Input: part model. Units: mm. Frame: model coordinates. A direction names the side the tool comes from. Coordinates: 2 decimals unless noted, no trailing zeros. Order: outer loops, then holes, each group sorted by start corner. A loop starts at its lowest first (then second) coordinate and runs counter-clockwise, first axis right, second up. Notation, with made-up numbers: (34.5, 3.5) -> (48.5, 3.5) arc R15 cw to (48.5, 29.5) -> close; hole circle Ø8 at (33, 87). An arc over 180 degrees is marked (long way). Answer as CSV lines item,"result".
from build123d import *

# Parameters (mm, degrees)
BOSS_EXTRUDE1_DEPTH      = 3
BOSS_EXTRUDE1_DEPTH_BACK = 3
SKETCH1_R                = 11
FILLET1_R                = 10


with BuildPart() as part:
    # Sketch1 → Boss-Extrude1 (new, two sides: drawn at the far end of the back side and taken through both)
    with BuildSketch(Plane(origin=(0, 0, 0), x_dir=(0, 0, -1), z_dir=(1, 0, 0)).offset(-BOSS_EXTRUDE1_DEPTH_BACK)):
        with BuildLine():
            Line((-5, -15.198684154), (-5, -80.198684154))
            ThreePointArc((-5, -80.198684154), (0, -111.397368307), (5, -80.198684154))
            Line((5, -80.198684154), (5, -15.198684154))
            ThreePointArc((5, -15.198684154), (0, 16), (-5, -15.198684154))
        make_face()
        Circle(SKETCH1_R, mode=Mode.SUBTRACT)
        with Locations((0, -95.397368307)):
            Circle(SKETCH1_R, mode=Mode.SUBTRACT)
    extrude(amount=BOSS_EXTRUDE1_DEPTH + BOSS_EXTRUDE1_DEPTH_BACK)

    # Fillet1
    fillet1_edges = [part.edges().sort_by_distance(p)[0] for p in [
        (0, -15.198684154, -5),
        (0, -80.198684154, -5),
        (0, -80.198684154, 5),
        (0, -15.198684154, 5),
    ]]
    fillet(fillet1_edges, radius=FILLET1_R)


solid = part.part
1. Contact query for a flat-ended pin moving along its axis: pin 1 (1.5 mm diameter, centred on x = -0.5, y = -43.5, fed in from -Z). Output: stop coordinate, or through.
Findings:
pin 1,"stops at z = -5"
2. Cut plane A-A (z = 0). Return the cut outline in (x, y), plus the area to 3 significant figures.
Findings:
outline,"(-3, -111.4) -> (3, -111.4) -> (3, -106.4) -> (-3, -106.4) -> close; (-3, -84.4) -> (3, -84.4) -> (3, -11) -> (-3, -11) -> close; (-3, 11) -> (3, 11) -> (3, 16) -> (-3, 16) -> close"
area,"500 mm2"
3. Ray query, line 1 along Y through (x, z) = (0.4, 0); line 2 along Y through (x, z) = (-0.6, -9); line 3 along Y through (x, z) = (-0.15, 9.5). Return the intervals inside material, ascending.
Findings:
line 1,"y = -111.4 to -106.4, -84.4 to -11, 11 to 16"
line 2,"y = -108.63 to -101.72, -89.07 to -82.16, -13.24 to -6.32, 6.32 to 13.23"
line 3,"y = -108.27 to -100.94, -89.85 to -82.52, -12.87 to -5.55, 5.55 to 12.87"
4. Cut plane D-D (x = -0.05). Return the cut outline in (y, z), plus the area to 3 significant figures.
Findings:
outline,"(-82.33, -9.23) arc R10 cw to (-74.16, -5) -> (-21.24, -5) arc R10 cw to (-13.07, -9.23) arc R16 ccw (long way) to (-13.07, 9.23) arc R10 cw to (-21.24, 5) -> (-74.16, 5) arc R10 cw to (-82.33, 9.23) arc R16 ccw (long way) to start; hole circle Ø22 at (-95.4, 0); hole circle Ø22 at (0, 0)"
area,"1,510 mm2"
5. Reachability of faces 3 (the face through (0.04, -16.58, -6.15)), 4 (the face through (-3, -43, 0)), 5 (the face through (0.04, -16.7, 6.09)) from +Z, -Z, +X, -X, +Y, -Y: full face, straight path, thin tool, end or side. Return the list, or none.
Findings:
face 3,"-Z, +X, -X"
face 4,"+Z, -Z, -X, +Y, -Y"
face 5,"+Z, +X, -X"
6. Cut plane B-B (y = 0). Return the cut outline in (x, z).
Findings:
outline,"(-3, -16) -> (3, -16) -> (3, -11) -> (-3, -11) -> close; (-3, 11) -> (3, 11) -> (3, 16) -> (-3, 16) -> close"
7. Mould query, pull axis Y, two halves, no side actions, for faces 1 (the face through (-0.04, -10.74, 2.38)), 2 (the face through (3, -43, 0)). Classes: released by +Y, released by -Y, zero draft, split by the parting line, or undercut.
Findings:
face 1,"undercut"
face 2,"zero draft"
8. Cut plane C-C (z = -7.5). Return the cut outline in (x, y).
Findings:
outline,"(-3, -109.53) -> (3, -109.53) -> (3, -103.44) -> (-3, -103.44) -> close; (-3, -87.35) -> (3, -87.35) -> (3, -80.77) -> (-3, -80.77) -> close; (-3, -14.62) -> (3, -14.62) -> (3, -8.05) -> (-3, -8.05) -> close; (-3, 8.05) -> (3, 8.05) -> (3, 14.13) -> (-3, 14.13) -> close"
